```python
from build123d import *

# Parameters (mm, degrees)
BOSS_EXTRUDE1_DEPTH = 15
FILLET1_R           = 5


with BuildPart() as part:
    # Sketch1 → Boss-Extrude1 (new body)
    with BuildSketch(Plane(origin=(0, 0, 0), x_dir=(1, 0, 0), z_dir=(0, 1, 0))):
        with BuildLine():
            Line((0, 0), (-296.420139667, 468.96320604))
            ThreePointArc((-296.420139667, 468.96320604), (-343.696667359, 508.335758373), (-405.074608149, 512.580323398))
            Line((-405.074608149, 512.580323398), (-1144.124532862, 328.861698046))
            ThreePointArc((-1144.124532862, 328.861698046), (-1198.779608041, 293.408896337), (-1220, 231.815281758))
            Line((-1220, 231.815281758), (-1220, -183.740597223))
            ThreePointArc((-1220, -183.740597223), (-1197.607828507, -246.804255176), (-1140.459500912, -281.625268252))
            Line((-1140.459500912, -281.625268252), (0, -520))
            Line((0, -520), (1140.459500912, -281.625268252))
            ThreePointArc((1140.459500912, -281.625268252), (1197.607828507, -246.804255176), (1220, -183.740597223))
            Line((1220, -183.740597223), (1220, 231.815281758))
            ThreePointArc((1220, 231.815281758), (1198.779608041, 293.408896337), (1144.124532862, 328.861698046))
            Line((1144.124532862, 328.861698046), (405.074608149, 512.580323398))
            ThreePointArc((405.074608149, 512.580323398), (343.696667359, 508.335758373), (296.420139667, 468.96320604))
            Line((296.420139667, 468.96320604), (0, 0))
        make_face()
    extrude(amount=BOSS_EXTRUDE1_DEPTH)

    # Fillet1
    fillet1_edges = [part.edges().sort_by_distance(p)[0] for p in [
        (-343.696667359, 15, -508.335758373),
        (343.696667359, 0, -508.335758373),
        (774.599570506, 0, -420.721010722),
        (1198.779608041, 0, -293.408896337),
        (1220, 0, -24.037342268),
        (1197.607828507, 0, 246.804255176),
        (570.229750456, 0, 400.812634126),
        (-570.229750456, 0, 400.812634126),
        (-1197.607828507, 0, 246.804255176),
        (-774.599570506, 15, -420.721010722),
        (-1220, 0, -24.037342268),
        (-1198.779608041, 0, -293.408896337),
        (-774.599570506, 0, -420.721010722),
        (-343.696667359, 0, -508.335758373),
        (-148.210069834, 0, -234.48160302),
        (148.210069834, 0, -234.48160302),
        (-1198.779608041, 15, -293.408896337),
        (-1220, 15, -24.037342268),
        (-1197.607828507, 15, 246.804255176),
        (-570.229750456, 15, 400.812634126),
        (570.229750456, 15, 400.812634126),
        (1197.607828507, 15, 246.804255176),
        (1220, 15, -24.037342268),
        (1198.779608041, 15, -293.408896337),
        (148.210069834, 15, -234.48160302),
        (774.599570506, 15, -420.721010722),
        (343.696667359, 15, -508.335758373),
        (-148.210069834, 15, -234.48160302),
    ]]
    fillet(fillet1_edges, radius=FILLET1_R)


solid = part.part
```
For this review, take the finished solid that the model builds, in its own axes (mm). A direction names the side the tool comes from. Round coordinates to 2 decimals unless told otherwise and drop trailing zeros. Write each loop counter-clockwise with the first axis right and the second up, starting at its lowest first coordinate (ties: lowest second). Pieces come first, ordered by that corner, then holes. Notation, with made-up numbers: (23.25, 3.5) -> (68.25, 3.5) arc R10 ccw to (68.25, 21.5) -> close; hole circle Ø9 at (-32, 70.25). An arc over 180 degrees is marked (long way). Use one line per item in the form item = value.
1) Tool access review of faces 5 (the flat face through (-146.135, 7.465, -231.199)), 6 (the cylindrical face through (-149.41, 13.5, -233.71)), 7 (the cylindrical face through (-1198.207, 7.465, 246.06)): name each direction out of +Z, -Z, +X, -X, +Y, -Y from which nothing blocks a thin tool from reaching the whole face with its end or side.
Found:
face_5 = -Z, +Y, -Y
face_6 = -Z, +Y
face_7 = +Z, -X, +Y, -Y
2) Mouldability with a two-part tool opening along X and no side actions: class faces 1 (the flat face through (-17, 0, -5)), 2 (the cylindrical face through (-342.89, 7.46, -508.01)), 3 (the cylindrical face through (577.921, 1.504, 397.748)), 4 (the cylindrical face through (145.198, 13.496, -227.047)) as +X half, -X half, draft (parallel to the pull), parting line (faces both ways), or undercut.
Found:
face_1 = draft
face_2 = undercut
face_3 = +X half
face_4 = undercut
3) Clearance check with flat-ended pins moving along their axes: pin 1 (5 mm diameter, centred on x = 318.5, y = 3, fed in from -Z); pin 2 (5 mm diameter, centred on x = 71, y = 8, fed in from +Z); pin 3 (5 mm diameter, centred on x = -173, y = 8.5, fed in from +Z). State where each tip first meets the part, or that it passes through.
Found:
pin_1 = -495.29
pin_2 = 505.68
pin_3 = 484.36
4) Take a section at A-A, the plane y = 7.5. Write out the cut boundary in (x, z), and give its area (3 significant figures).
Found:
outline = (-1220, -231.82) arc R100 ccw to (-1144.12, -328.86) -> (-405.07, -512.58) arc R100 ccw to (-296.42, -468.96) -> (0, 0) -> (296.42, -468.96) arc R100 ccw to (405.07, -512.58) -> (1144.12, -328.86) arc R100 ccw to (1220, -231.82) -> (1220, 183.74) arc R100 ccw to (1140.46, 281.63) -> (0, 520) -> (-1140.46, 281.63) arc R100 ccw to (-1220, 183.74) -> close
area = 1,870,000 mm2
5) To check wall thickness, follow L1, parallel to X at y = 5.25, z = -304; L2, parallel to X at y = 13.75, z = 78; L3, parallel to Z at x = 830, y = 3.25. State the ranges of each line that lie inside material, in increasing order. Write a range as from..to.
Found:
L1 = -1189.21..-192.15, 192.15..1189.21
L2 = -1218.31..1218.31
L3 = -406.62..346.19
